from build123d import *

# Parameters (mm, degrees)
F0_W           = 208.6787745357
F0_H           = 89.537139982
F1_DEPTH       = 109.8
F3_D           = 11
F3_CBORE_D     = 17.25
F3_CBORE_DEPTH = 10
F4_R           = 5
F5_SIZE        = 5


with BuildPart() as f1:
    # F0 (on Front) → F1 (new body)
    with BuildSketch(Plane.XZ):
        with Locations((9.4242058694, 10.4618463665)):
            Rectangle(F0_W, F0_H)
    extrude(amount=F1_DEPTH)

    # F3 (through all)
    with Locations(Plane.XY.offset(55.2304163575)):
        with Locations((-39.9151813984, -53.8)):
            CounterBoreHole(F3_D / 2, F3_CBORE_D / 2, F3_CBORE_DEPTH)

    # F4
    f4_edges = [f1.edges().sort_by_distance(p)[0] for p in [
        (113.763593, -54.9, 55.230416),
    ]]
    fillet(f4_edges, radius=F4_R)

    # F5
    f5_edges = [f1.edges().sort_by_distance(p)[0] for p in [
        (6.924206, 0, 55.230416),
    ]]
    chamfer(f5_edges, length=F5_SIZE)


solid = f1.part
Design review of the part built by this model. Coordinates are the model's own, in mm. A direction names the side the tool comes from. Give positions to 0.01 mm unless a question says otherwise; leave off trailing zeros. Loops run counter-clockwise (first coordinate to the right, second up) from the corner with the lowest first, then second, coordinate; pieces in that order, holes last. Notation, with made-up numbers: (46, -25.75) -> (78, -25.75) arc R17 cw to (78, -0.75) -> close; hole circle Ø7 at (74, -33). An arc over 180 degrees is marked (long way). One line per question, with ' | ' between items. Start each with the question number.
(1) Insertion check: P1, Ø6.5, axis at x = -39.92, y = -53.8, coming from the -Z side; P2, Ø15.5, axis at x = -39.92, y = -53.8, coming from the +Z side. Each pin has a flat end and moves straight along its axis. Give the tip position at first contact, or say it passes through.
(2) We need section B-B (x = -40). State the section outline as (y, z) points.
(3) For line 1 (X direction, y = -53, z = 6); line 2 (Y direction, x = -37, z = 0); line 3 (X direction, y = -53, z = 52), list the stretches that pass through material, from the lowest coordinate up.
(4) Draft analysis for pull direction Y (two halves, no side actions). For faces 3 (the face through (5.498, -2.465, 52.695)), 4 (the face through (-34, -54, 45.23)), 5 (the face through (8, -54, -34.307)), 6 (the face through (-38.72, -59.17, 4.91)), state which applies: +Y half, -Y half, draft (parallel to the pull), parting line (faces both ways), or undercut.
(5) We need section A-A (y = -53.8). State the section outline as (x, z) points.
(6) For faces 1 (the face through (-48.53, -53.42, 50.3)), 2 (the face through (5, 0, 9)), list the 3-axis set-ups (+Z, -Z, +X, -X, +Y, -Y) from which the entire face can be reached by the end or side of a thin tool; tool diameter is ignored.
The answers:
1) P1: passes through | P2: stops at z = 45.23
2) outline: (-109.8, -34.31) -> (-59.3, -34.31) -> (-59.3, 45.23) -> (-62.42, 45.23) -> (-62.42, 55.23) -> (-109.8, 55.23) -> close; (-48.3, -34.31) -> (0, -34.31) -> (0, 50.23) -> (-5, 55.23) -> (-45.18, 55.23) -> (-45.18, 45.23) -> (-48.3, 45.23) -> close
3) line 1: x = -94.92 to -45.36, -34.47 to 113.76 | line 2: y = -109.8 to -58.46, -49.14 to 0 | line 3: x = -94.92 to -48.5, -31.33 to 113.44
4) face 3: +Y half | face 4: undercut | face 5: draft | face 6: undercut
5) outline: (-94.92, -34.31) -> (-45.42, -34.31) -> (-45.42, 45.23) -> (-48.54, 45.23) -> (-48.54, 55.23) -> (-94.92, 55.23) -> close; (-34.42, -34.31) -> (113.76, -34.31) -> (113.76, 50.23) arc R5 ccw to (108.76, 55.23) -> (-31.29, 55.23) -> (-31.29, 45.23) -> (-34.42, 45.23) -> close
6) face 1: +Z | face 2: +Z, -Z, +X, -X, +Y
